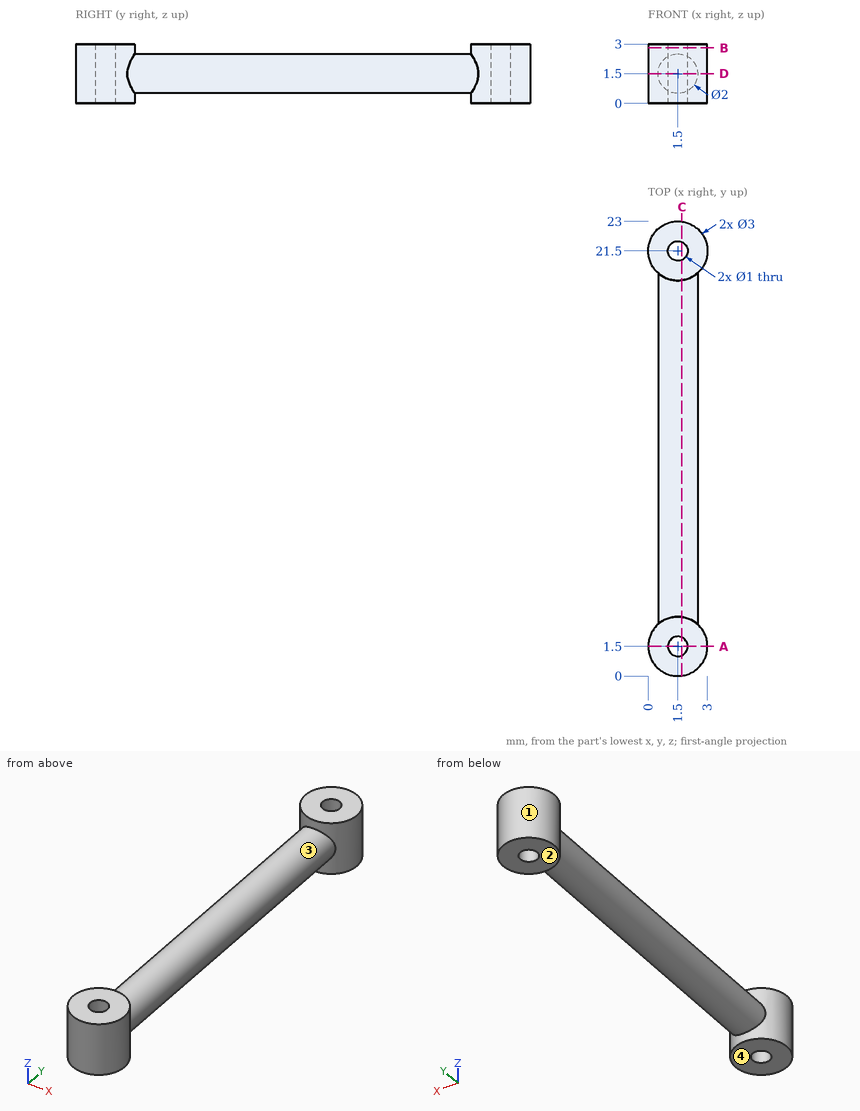
The drawing under review shows one solid part. Ordinate dimensions are in mm from its lowest x, y, z. A direction names the side the tool comes from. Round coordinates to 2 decimals unless told otherwise and drop trailing zeros. Loops run counter-clockwise (first coordinate to the right, second up) from the corner with the lowest first, then second, coordinate; pieces in that order, holes last. Notation, with made-up numbers: M 30.5,29 L 40.5,29 A21 ccw 40.5,64 Z; hole C 1,1 d2. An arc over 180 degrees is marked long. Answer as CSV lines item,"result". Start each with the question number.
Item 1: Mouldability with a two-part tool opening along Y and no side actions: class the marked faces 1 and 2 as released by +Y, released by -Y, zero draft, split by the parting line, or undercut.
Item 2: Insertion check: P1, Ø1.5, axis at y = 12.5, z = 2, coming from the -X side. The pin has a flat end and moves straight along its axis. Give the tip position at first contact, or say it passes through.
Item 3: Consider section D-D (z = 1.5). Write out the cut boundary in (x, y), then the cut area to 3 significant figures.
Item 4: Consider section A-A (y = 1.5). Write out the cut boundary in (x, z).
Item 5: Consider section B-B (z = 2.8). Write out the cut boundary in (x, y), then the cut area to 3 significant figures.
Item 6: Wall thickness on line 1 (Y direction, x = 1.5, z = 2.45); line 2 (Z direction, x = 1.6, y = 11.75); line 3 (X direction, y = 4.25, z = 1.55): over which ranges is each line inside the solid? List them lowest first. Write a range as [from, to].
Item 7: For the marked faces 3 and 4, list the 3-axis set-ups (+Z, -Z, +X, -X, +Y, -Y) from which the entire face can be reached by the end or side of a thin tool; tool diameter is ignored.
Item 8: Consider section C-C (x = 1.7). Write out the cut boundary in (y, z).
Answer:
1,face 1,"undercut"
1,face 2,"zero draft"
2,P1,"stops at x = 0.5"
3,outline,"M 0.5,2.62 A1.5 ccw long 2.5,2.62 L 2.5,20.38 A1.5 ccw long 0.5,20.38 Z; hole C 1.5,1.5 d1; hole C 1.5,21.5 d1"
3,area,"47.0 mm^2"
4,outline,"M 0,0 L 1,0 L 1,3 L 0,3 Z; M 2,0 L 3,0 L 3,3 L 2,3 Z"
5,outline,"C 1.5,1.5 d3; C 1.5,21.5 d3; hole C 1.5,1.5 d1; hole C 1.5,21.5 d1"
5,area,"12.6 mm^2"
6,line 1,"y = [0, 1], [2, 21], [22, 23]"
6,line 2,"z = [0.51, 2.49]"
6,line 3,"x = [0.5, 2.5]"
7,face 3,"none"
7,face 4,"-Z, +X, -X, +Y, -Y"
8,outline,"M 0.01,0 L 1.04,0 L 1.04,3 L 0.01,3 Z; M 1.96,0 L 2.99,0 L 2.99,0.52 L 20.01,0.52 L 20.01,0 L 21.04,0 L 21.04,3 L 20.01,3 L 20.01,2.48 L 2.99,2.48 L 2.99,3 L 1.96,3 Z; M 21.96,0 L 22.99,0 L 22.99,3 L 21.96,3 Z"
